Drawing for the job (mm, zero at the part's lowest x, y, z). Give positions to 0.01 mm unless a question says otherwise; leave off trailing zeros. Order: outer loops, then holes, each group sorted by start corner. A loop starts at its lowest first (then second) coordinate and runs counter-clockwise, first axis right, second up. Notation, with made-up numbers: (33, 37) - (60, 37) arc R30 ccw to (60, 74) - close; hole circle Ø1 at (36, 14). An arc over 180 degrees is marked (long way). Use a Markdown table: item, result.
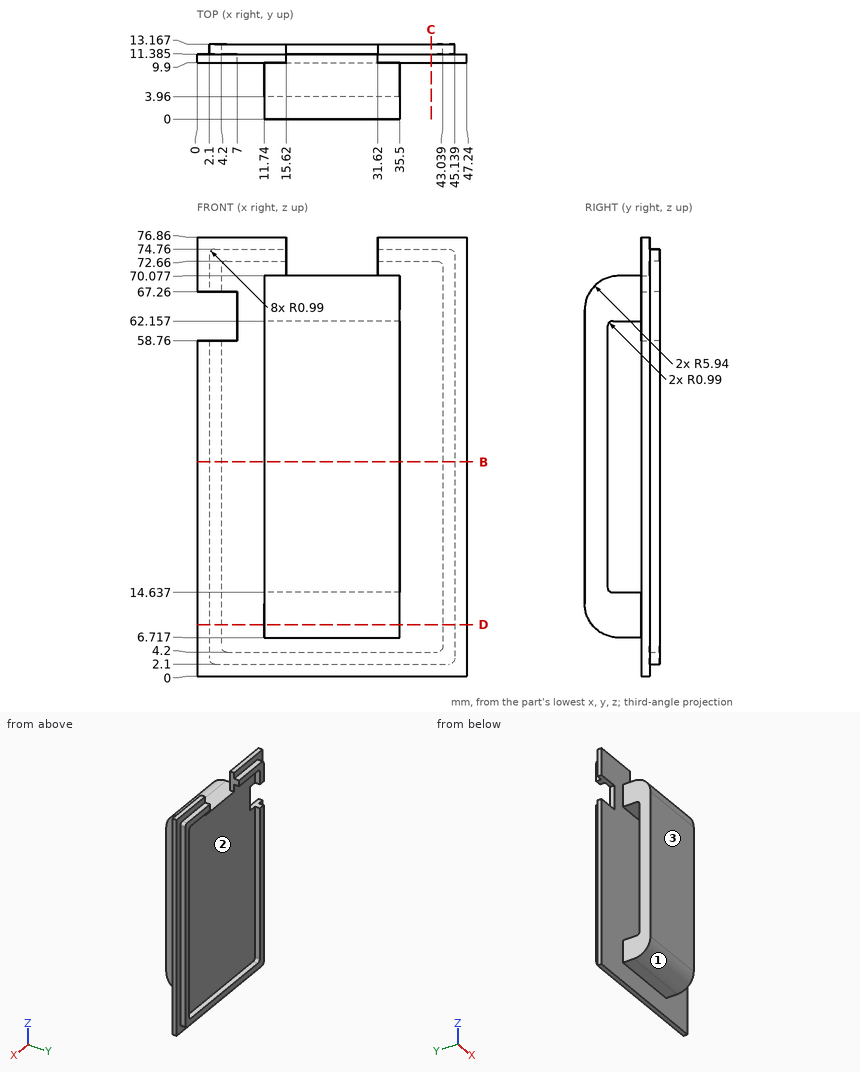
1) Slice it at C-C (x = 41). Write the cut outline in (y, z) (1 decimal).
Computed:
| item | result |
|---|---|
| outline | (9.9, 0) - (11.4, 0) - (11.4, 2.1) - (13.2, 2.1) - (13.2, 4.2) - (11.4, 4.2) - (11.4, 72.7) - (13.2, 72.7) - (13.2, 74.8) - (11.4, 74.8) - (11.4, 76.9) - (9.9, 76.9) - close |
2) Pin check, flat tips, straight feed: P1, Ø1.4, axis at x = 36.5, y = 12, coming from the -Z side; P2, Ø0.9, axis at x = 8.5, y = 12.5, coming from the +Z side; P3, Ø1, axis at y = 5, z = 67, coming from the +X side; P4, Ø2.5, axis at x = 29, y = 8.5, coming from the -Z side. Stop position of each tip, or through.
Computed:
| item | result |
|---|---|
| P1 | stops at z = 0 |
| P2 | stops at z = 74.76 |
| P3 | stops at x = 35.5 |
| P4 | stops at z = 6.72 |
3) Slice it at B-B (z = 37.5). Write the cut outline in (x, y) (1 decimal).
Computed:
| item | result |
|---|---|
| outline | (0, 9.9) - (47.2, 9.9) - (47.2, 11.4) - (45.1, 11.4) - (45.1, 13.2) - (43, 13.2) - (43, 11.4) - (4.2, 11.4) - (4.2, 13.2) - (2.1, 13.2) - (2.1, 11.4) - (0, 11.4) - close; (11.7, 0) - (35.5, 0) - (35.5, 4) - (11.7, 4) - close |
4) Slice it at D-D (z = 9). Write the cut outline in (x, y) (1 decimal), and give its area (3 significant figures).
Computed:
| item | result |
|---|---|
| outline | (0, 9.9) - (11.7, 9.9) - (11.7, 1.3) - (35.5, 1.3) - (35.5, 9.9) - (47.2, 9.9) - (47.2, 11.4) - (45.1, 11.4) - (45.1, 13.2) - (43, 13.2) - (43, 11.4) - (4.2, 11.4) - (4.2, 13.2) - (2.1, 13.2) - (2.1, 11.4) - (0, 11.4) - close |
| area | 283 mm² |
5) Two-plate mould, pull along Z, no slides. Class the marked faces 1, 2 and 3: +Z half, -Z half, draft (parallel to the pull), parting line (faces both ways), or undercut.
Computed:
| item | result |
|---|---|
| face 1 | -Z half |
| face 2 | undercut |
| face 3 | draft |
6) Wall check: line 1 (Z direction, x = 28, y = 7.25); line 2 (Y direction, x = 22.5, z = 49) (1 decimal); line 3 (X direction, y = 12.5, z = 53). Give the ranges that are in metal, low to high. Write a range as from..to.
Computed:
| item | result |
|---|---|
| line 1 | z = 6.72..14.64, 62.16..70.08 |
| line 2 | y = 0..4, 9.9..11.4 |
| line 3 | x = 2.1..4.2, 43.04..45.14 |
